```python
from build123d import *

# Parameters (mm, degrees)
F_5_16_CLEARANCE_HOLE1_D         = 8.4328
CIRPATTERN1_COUNT                = 12
F_1_2_0_5_DIAMETER_HOLE1_D       = 12.7
F_1_1_5_DIAMETER_HOLE1_D         = 38.1
F_1_1_5_DIAMETER_HOLE1_DEPTH     = 19.05
CIRPATTERN2_COUNT                = 6
CIRPATTERN3_COUNT                = 2
F_1_8_0_125_DIAMETER_HOLE1_D     = 3.175
F_1_8_0_125_DIAMETER_HOLE1_DEPTH = 6.35
F_1_8_0_125_DIAMETER_HOLE1_TIP   = 0.953866233


with BuildPart() as part:
    # Sketch1 → Revolve1 (revolve)
    with BuildSketch(Plane.XY, mode=Mode.PRIVATE) as revolve1_sk:
        Polygon((-55.9435, 0), (-88.9, 0), (-88.9, 38.1), (-50.8, 38.1), (-31.75, 57.15), (-12.573, 57.15), (-12.573, 55.118), (-9.525, 55.118), (-9.525, 57.15), (-6.35, 57.15), (-6.35, 53.975), (-8.382, 53.975), (-8.382, 50.927), (-6.35, 50.927), (-6.35, 31.75), (-31.75, 31.75), (-31.75, 19.05), (-50.8, 19.05), (-50.8, 0), (-52.3875, 0), (-52.3875, 2.54), (-55.9435, 2.54), align=None)
    revolve(revolve1_sk.sketch.rotate(Axis((0, 0, 0), (0, 1, 0)), 270), axis=Axis((0, 0, 0), (0, 1, 0)))

    # 5/16 Clearance Hole1 (through all)
    with Locations(Plane(origin=(0, 38.1, 0), x_dir=(1, 0, 0), z_dir=(0, 1, 0))):
        with Locations((-73.603547963, -19.722011237)):
            f_5_16_clearance_hole1 = Hole(F_5_16_CLEARANCE_HOLE1_D / 2)

    # CirPattern1: 5/16 Clearance Hole1 ×12 about axis
    cirpattern1_axis = Axis((0, 0, 0), (0, 1, 0))
    for i in range(1, CIRPATTERN1_COUNT):
        add(f_5_16_clearance_hole1.rotate(cirpattern1_axis, i * 360 / CIRPATTERN1_COUNT), mode=Mode.SUBTRACT)

    # 1/2 (0.5) Diameter Hole1 (through all)
    with Locations(Plane(origin=(0, 57.15, 0), x_dir=(1, 0, 0), z_dir=(0, 1, 0))):
        with Locations((0, 0)):
            Hole(F_1_2_0_5_DIAMETER_HOLE1_D / 2)

    # Sketch11 → 1/2 NPT Tapped Hole1 (revolve, cut)
    with BuildSketch(Plane(origin=(41.275, 47.625, 0), x_dir=(-0.707106781186546, 0.707106781186549, 0), z_dir=(0, 0, 1))):
        Polygon((0, 0), (0, 125.723585695), (8.9281, 125.723585695), (8.9281, 13.462), (9.479726792, 13.462), (9.8827971, 0), align=None)
    revolve(axis=Axis((45.765128061, 52.115128061, 0), (-0.707106781186549, -0.707106781186546, 0)), mode=Mode.SUBTRACT)

    # 1 (1.5) Diameter Hole1
    with Locations(Plane(origin=(0, 57.15, 0), x_dir=(1, 0, 0), z_dir=(0, 1, 0))):
        with Locations((-23.8125, -41.244459855)):
            f_1_1_5_diameter_hole1 = Hole(F_1_1_5_DIAMETER_HOLE1_D / 2, depth=F_1_1_5_DIAMETER_HOLE1_DEPTH)

    # Sketch19 → 3/8 NPT Tapped Hole1 (revolve, cut)
    with BuildSketch(Plane(origin=(-23.8125, 38.1, 41.244459855), x_dir=(0, 0, 1), z_dir=(1, 0, 0))):
        Polygon((0, 0), (0, 26.640582582), (7.1374, 22.352), (7.1374, 10.414), (7.653732494, 10.414), (7.9655416, 0), align=None)
    f_3_8_npt_tapped_hole1 = revolve(axis=Axis((-23.8125, 44.45, 41.244459855), (0, -1, 0)), mode=Mode.SUBTRACT)

    # Sketch21 → 1/4 (0.25) Diameter Hole1 (revolve, cut)
    with BuildSketch(Plane(origin=(21.997045256, 57.15, -12.7), x_dir=(0, 0, 1), z_dir=(1, 0, 0))):
        Polygon((0, 0), (0, 17.909732465), (3.175, 16.002), (3.175, 0), align=None)
    f_1_4_0_25_diameter_hole1 = revolve(axis=Axis((21.997045256, 63.5, -12.7), (0, -1, 0)), mode=Mode.SUBTRACT)

    # CirPattern2: 1/4 (0.25) Diameter Hole1 ×6 about axis
    cirpattern2_axis = Axis((0, 0, 0), (0, 1, 0))
    for i in range(1, CIRPATTERN2_COUNT):
        add(f_1_4_0_25_diameter_hole1.rotate(cirpattern2_axis, i * 360 / CIRPATTERN2_COUNT), mode=Mode.SUBTRACT)

    # CirPattern3: 1 (1.5) Diameter Hole1, 3/8 NPT Tapped Hole1 ×2 about axis
    cirpattern3_axis = Axis((0, 0, 0), (0, 1, 0))
    add([f_1_1_5_diameter_hole1.rotate(cirpattern3_axis, i * 360 / CIRPATTERN3_COUNT) for i in range(1, CIRPATTERN3_COUNT)], mode=Mode.SUBTRACT)
    add([f_3_8_npt_tapped_hole1.rotate(cirpattern3_axis, i * 360 / CIRPATTERN3_COUNT) for i in range(1, CIRPATTERN3_COUNT)], mode=Mode.SUBTRACT)

    # 1/8 (0.125) Diameter Hole1
    with Locations(Plane(origin=(0, 19.05, 0), x_dir=(-1, 0, 0), z_dir=(0, -1, 0))):
        with Locations((0, -44.45)):
            Hole(F_1_8_0_125_DIAMETER_HOLE1_D / 2, depth=F_1_8_0_125_DIAMETER_HOLE1_DEPTH)
            with Locations((0, 0, -(F_1_8_0_125_DIAMETER_HOLE1_DEPTH + F_1_8_0_125_DIAMETER_HOLE1_TIP / 2))):  # 118° drill point
                Cone(0, F_1_8_0_125_DIAMETER_HOLE1_D / 2, F_1_8_0_125_DIAMETER_HOLE1_TIP, mode=Mode.SUBTRACT)


solid = part.part
```
Source: CAD feature listing. Evaluate the final solid. Frame: model axes, mm. A direction names the side the tool comes from. Coordinates: 2 decimals unless noted, no trailing zeros. Loops run counter-clockwise (first coordinate to the right, second up) from the corner with the lowest first, then second, coordinate; pieces in that order, holes last. Notation, with made-up numbers: M 45,39 L 73,39 A14 ccw 73,49 Z; hole C -24,3.25 d11. An arc over 180 degrees is marked long. Put each result on its own line as item: value. Start each with the question number.
1) Reachability of faces 1 (the face through (58, 0, -1)), 2 (the face through (21.9, 19.05, -23.3)), 3 (the face through (27, 27.686, -48)), 4 (the face through (-69.39, 18.78, 19.54)), 5 (the face through (-6, 53.975, 3)) from +Z, -Z, +X, -X, +Y, -Y: full face, straight path, thin tool, end or side. Return the list, or none.
2) Cut plane B-B on x = -73.5. Return the cut outline in (y, z).
3) Contact query for flat-ended pins moving along their axis: pin 1 Ø4 at (x, y) = (35.5, 46) entering from -Z; pin 2 Ø1.9 at (x, z) = (0, 44.45) entering from -Y; pin 3 Ø5 at (x, z) = (37.5, -14) entering from +Y; pin 4 Ø5 at (x, z) = (0, -2.5) entering from -Y. Output: stop coordinate, or through.
4) Cut plane C-C on x = 64. Return the cut outline in (y, z), then the cut area to 3 significant figures.
5) Ray query, L1, parallel to X at y = 55.5, z = 0 (3 decimals); L2, parallel to X at y = 3.5, z = 56.5; L3, parallel to X at y = 16.5, z = 75.5. Return the intervals inside material, ascending. Write a range as from..to.
6) Cut plane D-D on z = -2.5. Give the number of separate pieces and of enclosed holes in the cut face, then the cut area to 3 significant figures.
7) Cut plane A-A on z = -73. Return the cut outline in (x, y) (3 decimals).
8) Pull-direction query (Z, two-part tool) for faces 6 (the face through (6.2, 57.15, -2)), 7 (the face through (-18.9, 49.3, -13.4)); classes: pulls with the +Z half, pulls with the -Z half, needs draft (parallel to the pull), parting line crosses it, or undercut.
The answers:
1. face 1: +Z, -Z, +X, -X, -Y
1. face 2: -Y
1. face 3: +Y
1. face 4: +Y, -Y
1. face 5: none
2. outline: M 0,-50.01 L 38.1,-50.01 L 38.1,-23.94 L 0,-23.94 Z; M 0,-15.51 L 38.1,-15.51 L 38.1,15.51 L 0,15.51 Z; M 0,23.94 L 38.1,23.94 L 38.1,50.01 L 0,50.01 Z
3. pin 1: stops at z = -26.64
3. pin 2: stops at y = 25.78
3. pin 3: stops at y = 51.37
3. pin 4: passes through
4. outline: M 0,-61.7 L 38.1,-61.7 L 38.1,61.7 L 0,61.7 Z
4. area: 4,700 mm²
5. L1: x = -33.4..-12.573, -9.525..-6.35, 6.35..9.525, 12.573..33.4
5. L2: x = -68.64..-57.19, -50.58..50.58, 57.19..68.64
5. L3: x = -46.94..-23.49, -15.96..15.96, 23.49..46.94
6. separate pieces: 3
6. enclosed holes: 0
6. area: 4,840 mm²
7. outline: M -50.737,0 L -23.895,0 L -23.895,38.1 L -50.737,38.1 Z; M -15.549,0 L 15.549,0 L 15.549,38.1 L -15.549,38.1 Z; M 23.895,0 L 50.737,0 L 50.737,38.1 L 23.895,38.1 Z
8. face 6: needs draft
8. face 7: undercut
